from build123d import *

# Parameters (mm, degrees)
SKETCH_1_W           = 5
SKETCH_1_H           = 8
EXTRUDE_1_DEPTH      = 5.2
EXTRUDE_1_2_DEPTH    = 5.2
EXTRUDE_1_3_DEPTH    = 5.2
EXTRUDE_1_4_DEPTH    = 5.2
SKETCH_2_W           = 3.1
SKETCH_2_H           = 5.8
EXTRUDE_2_DEPTH      = 5
EXTRUDE_3_DEPTH      = 2
EXTRUDE_3_DEPTH_BACK = 1
SKETCH_3_W           = 2.6
SKETCH_3_H           = 0.6
FILLET_1_R           = 0.75


with BuildPart() as part:
    # Sketch 1 → Extrude 1 (new body)
    with BuildSketch(Plane.XY):
        with Locations((2.5, 0.600266138)):
            Rectangle(SKETCH_1_W, SKETCH_1_H)
    extrude(amount=EXTRUDE_1_DEPTH)



with BuildPart() as body_2:
    # Sketch 1 → Extrude 1 2 (new body)
    with BuildSketch(Plane.XY):
        with Locations((-5.1, 0.600266138)):
            Rectangle(SKETCH_1_W, SKETCH_1_H)
    extrude(amount=EXTRUDE_1_2_DEPTH)


with BuildPart() as body_3:
    # Sketch 1 → Extrude 1 3 (new body)
    with BuildSketch(Plane.XY):
        with Locations((10.1, 0.600266138)):
            Rectangle(SKETCH_1_W, SKETCH_1_H)
    extrude(amount=EXTRUDE_1_3_DEPTH)


with BuildPart() as body_4:
    # Sketch 1 → Extrude 1 4 (new body)
    with BuildSketch(Plane.XY):
        with Locations((17.7, 0.600266138)):
            Rectangle(SKETCH_1_W, SKETCH_1_H)
    extrude(amount=EXTRUDE_1_4_DEPTH)


with BuildPart() as part_1:
    add(part.part)

    add(body_2.part)  # Extrude 2 merges body 2

    add(body_3.part)  # Extrude 2 merges body 3

    add(body_4.part)  # Extrude 2 merges body 4
    # Sketch 2 → Extrude 2 (add)
    with BuildSketch(Plane(origin=(0, 0, 0), x_dir=(-1, 0, 0), z_dir=(0, 0, -1))):
        with Locations((-17.7, 0.600266138)):
            Rectangle(SKETCH_2_W, SKETCH_2_H)
        with Locations((-10.1, 0.600266138)):
            Rectangle(SKETCH_2_W, SKETCH_2_H)
        with Locations((-2.5, 0.600266138)):
            Rectangle(SKETCH_2_W, SKETCH_2_H)
        with Locations((5.1, 0.600266138)):
            Rectangle(SKETCH_2_W, SKETCH_2_H)
    extrude(amount=EXTRUDE_2_DEPTH)

    # Sketch 3 → Extrude 3 (add, two sides: drawn at the far end of the back side and taken through both)
    with BuildSketch(Plane(origin=(0, 0, 0), x_dir=(1, 0, 0), z_dir=(0, 1, 0)).offset(-EXTRUDE_3_DEPTH_BACK)):
        with Locations((-1.3, -0.3)):
            Rectangle(SKETCH_3_W, SKETCH_3_H)
        with Locations((6.3, -0.3)):
            Rectangle(SKETCH_3_W, SKETCH_3_H)
        with Locations((13.9, -0.3)):
            Rectangle(SKETCH_3_W, SKETCH_3_H)
    extrude(amount=EXTRUDE_3_DEPTH + EXTRUDE_3_DEPTH_BACK)

    # Fillet 1
    fillet_1_edges = [part_1.edges().sort_by_distance(p)[0] for p in [
        (16.15, 3.500266138, -2.5),
        (19.25, 3.500266138, -2.5),
        (19.25, -2.299733862, -2.5),
        (16.15, -2.299733862, -2.5),
        (17.7, 3.500266138, -5),
        (19.25, 0.600266138, -5),
        (17.7, -2.299733862, -5),
        (16.15, 0.600266138, -5),
        (-6.65, 3.500266138, -2.5),
        (-3.55, 3.500266138, -2.5),
        (-3.55, -2.299733862, -2.5),
        (-6.65, -2.299733862, -2.5),
        (-5.1, 3.500266138, -5),
        (-3.55, 0.600266138, -5),
        (-5.1, -2.299733862, -5),
        (-6.65, 0.600266138, -5),
        (0.95, 3.500266138, -2.5),
        (4.05, 3.500266138, -2.5),
        (4.05, -2.299733862, -2.5),
        (0.95, -2.299733862, -2.5),
        (2.5, 3.500266138, -5),
        (4.05, 0.600266138, -5),
        (2.5, -2.299733862, -5),
        (0.95, 0.600266138, -5),
        (8.55, 3.500266138, -2.5),
        (11.65, 3.500266138, -2.5),
        (11.65, -2.299733862, -2.5),
        (8.55, -2.299733862, -2.5),
        (10.1, 3.500266138, -5),
        (11.65, 0.600266138, -5),
        (10.1, -2.299733862, -5),
        (8.55, 0.600266138, -5),
    ]]
    fillet(fillet_1_edges, radius=FILLET_1_R)


solid = part_1.part
Input: part model. Units: mm. Frame: model coordinates. A direction names the side the tool comes from. Give positions to 0.01 mm unless a question says otherwise; leave off trailing zeros. Order: outer loops, then holes, each group sorted by start corner. A loop starts at its lowest first (then second) coordinate and runs counter-clockwise, first axis right, second up.
Q1. Section A-A on z = 4.25. Output: boundary loops of the cut face in (x, y), and give its area (3 significant figures).
Checked values:
outline: (-7.6, -3.4) - (-2.6, -3.4) - (-2.6, 4.6) - (-7.6, 4.6) - close; (0, -3.4) - (5, -3.4) - (5, 4.6) - (0, 4.6) - close; (7.6, -3.4) - (12.6, -3.4) - (12.6, 4.6) - (7.6, 4.6) - close; (15.2, -3.4) - (20.2, -3.4) - (20.2, 4.6) - (15.2, 4.6) - close
area: 160 mm2
Q2. Section B-B on x = -5. Output: boundary loops of the cut face in (y, z).
Checked values:
outline: (-3.4, 0) - (-2.3, 0) - (-2.3, -4.25) arc R0.75 ccw to (-1.55, -5) - (2.75, -5) arc R0.75 ccw to (3.5, -4.25) - (3.5, 0) - (4.6, 0) - (4.6, 5.2) - (-3.4, 5.2) - close
Q3. Ray query, probe 1 along X at (y, z) = (1, 4.75); probe 2 along X at (y, z) = (-1.5, -2.25); probe 3 along Z at (x, y) = (7, 1). Return the intervals inside material, ascending.
Checked values:
probe 1: x = -7.6 to -2.6, 0 to 5, 7.6 to 12.6, 15.2 to 20.2
probe 2: x = -6.65 to -3.55, 0.95 to 4.05, 8.55 to 11.65, 16.15 to 19.25
probe 3: z = 0 to 0.6
Q4. Set-up query: faces 5 (the flat face through (-3.55, 1, -2)), 6 (the flat face through (10, -2.3, -2)), 7 (the flat face through (18, 3.5, -2)). Return all of +Z, -Z, +X, -X, +Y, -Y with unobstructed straight access to the full face (end or side cutting, diameter ignored); none if empty.
Checked values:
face 5: -Z, +Y, -Y
face 6: -Z, +X, -X, -Y
face 7: -Z, +X, -X, +Y
Q5. Draft query along X for faces 1 (the flat face through (-5, -2.3, -2)), 2 (the flat face through (14, 0, 0.6)), 3 (the flat face through (20.2, 1, 3)), 4 (the flat face through (11.65, 1, -2)). Return one class per face: +X half, -X half, draft (parallel to the pull), parting line (faces both ways), or undercut.
Checked values:
face 1: draft
face 2: undercut
face 3: +X half
face 4: undercut
Q6. Contact query for flat-ended pins moving along their axis: pin 1 Ø2 at (x, z) = (12, -3) entering from +Y; pin 2 Ø3 at (x, z) = (5, -2.5) entering from -Y; pin 3 Ø1 at (x, y) = (0, -2) entering from -Z. Output: stop coordinate, or through.
Checked values:
pin 1: stops at y = 3.49
pin 2: stops at y = -2.27
pin 3: stops at z = 0
Q7. Section C-C on z = -2.75. State how many separate pieces and enclosed holes the cut face has, and give its area (3 significant figures).
Checked values:
separate pieces: 4
enclosed holes: 0
area: 70.0 mm2
